Check sheet for the modelled part. Datum: model origin and axes. Units: mm. A direction names the side the tool comes from. Round coordinates to 2 decimals unless told otherwise and drop trailing zeros. Order: outer loops, then holes, each group sorted by start corner. A loop starts at its lowest first (then second) coordinate and runs counter-clockwise, first axis right, second up. Notation, with made-up numbers: (18, 47) -> (64, 47) arc R10 cw to (64, 66) -> close; hole circle Ø11 at (70.25, 52.5). An arc over 180 degrees is marked (long way). Answer in a Markdown table with one row per item.
```python
from build123d import *

# Parameters (mm, degrees)
F0_W     = 186
F0_H     = 44
F1_DEPTH = 15
F2_W     = 186
F2_H     = 44
F3_DEPTH = 2
F4_R     = 12
F5_SIZE  = 1.5


with BuildPart() as f1:
    # F0 (on Top) → F1 (new body)
    with BuildSketch(Plane.XY):
        with Locations((91, 20)):
            Rectangle(F0_W, F0_H)
        with BuildLine():
            ThreePointArc((122, 30), (124.9289321881, 37.0710678119), (132, 40))
            Line((132, 40), (172, 40))
            ThreePointArc((172, 40), (179.0710678119, 37.0710678119), (182, 30))
            Line((182, 30), (182, 10))
            ThreePointArc((182, 10), (179.0710678119, 2.9289321881), (172, 0))
            Line((172, 0), (132, 0))
            ThreePointArc((132, 0), (124.9289321881, 2.9289321881), (122, 10))
            Line((122, 10), (122, 30))
        make_face(mode=Mode.SUBTRACT)
        with BuildLine():
            Line((110, 0), (10, 0))
            ThreePointArc((10, 0), (2.9289321881, 2.9289321881), (0, 10))
            Line((0, 10), (0, 30))
            ThreePointArc((0, 30), (2.9289321881, 37.0710678119), (10, 40))
            Line((10, 40), (110, 40))
            ThreePointArc((110, 40), (117.0710678119, 37.0710678119), (120, 30))
            Line((120, 30), (120, 10))
            ThreePointArc((120, 10), (117.0710678119, 2.9289321881), (110, 0))
        make_face(mode=Mode.SUBTRACT)
    extrude(amount=F1_DEPTH)

    # F2 (on face) → F3 (join)
    with BuildSketch(Plane(origin=(0, 0, 0), x_dir=(1, 0, 0), z_dir=(0, 0, -1))):
        with Locations((91, -20)):
            Rectangle(F2_W, F2_H)
    extrude(amount=-F3_DEPTH)

    # F4
    f4_edges = [f1.edges().sort_by_distance(p)[0] for p in [
        (-2, -2, 7.5),
        (-2, 42, 7.5),
        (184, -2, 7.5),
        (184, 42, 7.5),
    ]]
    fillet(f4_edges, radius=F4_R)

    # F5
    f5_edges = [f1.edges().sort_by_distance(p)[0] for p in [
        (60, 0, 2),
        (117.071068, 2.928932, 2),
        (120, 20, 2),
        (117.071068, 37.071068, 2),
        (60, 40, 2),
        (2.928932, 37.071068, 2),
        (0, 20, 2),
        (2.928932, 2.928932, 2),
        (152, 0, 2),
        (179.071068, 2.928932, 2),
        (182, 20, 2),
        (179.071068, 37.071068, 2),
        (152, 40, 2),
        (124.928932, 37.071068, 2),
        (122, 20, 2),
        (124.928932, 2.928932, 2),
        (180.485281, 1.514719, 0),
    ]]
    chamfer(f5_edges, length=F5_SIZE)


solid = f1.part
```
(1) Scan lines: probe 1 along X at (y, z) = (10, 7.75); probe 2 along Y at (x, z) = (78.5, 10.25); probe 3 along X at (y, z) = (10.5, 3). Record each from-to range of solid material in increasing order. Write a range as from..to.
Solutions:
| item | result |
|---|---|
| probe 1 | -2..0, 120..122, 182..184 |
| probe 2 | -2..0, 40..42 |
| probe 3 | -2..0.5, 119.5..122.5, 181.5..184 |
(2) Depth check by flat-ended pin: pin 1 Ø18.5 at (x, y) = (73.5, 27.5) entering from +Z. Enter the tip coordinate at first touch or a pass-through.
Solutions:
| item | result |
|---|---|
| pin 1 | z = 2 |
(3) Section check C-C on x = 15.5. Record the boundary of the cut face in (y, z), plus the area to 3 significant figures.
Solutions:
| item | result |
|---|---|
| outline | (-2, 1.5) -> (-0.5, 0) -> (40.5, 0) -> (42, 1.5) -> (42, 15) -> (40, 15) -> (40, 3.5) -> (38.5, 2) -> (1.5, 2) -> (0, 3.5) -> (0, 15) -> (-2, 15) -> close |
| area | 140 mm^2 |
(4) Tool access check on faces 4 (the flat face through (-2, 20, 8)), 5 (the cylindrical face through (3.01, 2.85, 9.17)). Record the directions out of +Z, -Z, +X, -X, +Y, -Y that give a thin tool (end or side, any length) a straight path to the whole face; none if there is none.
Solutions:
| item | result |
|---|---|
| face 4 | +Z, -Z, -X, +Y, -Y |
| face 5 | +Z |
(5) Section check B-B on y = 14.5. Record the boundary of the cut face in (x, z).
Solutions:
| item | result |
|---|---|
| outline | (-2, 1.5) -> (-0.5, 0) -> (182.5, 0) -> (184, 1.5) -> (184, 15) -> (182, 15) -> (182, 3.5) -> (180.5, 2) -> (123.5, 2) -> (122, 3.5) -> (122, 15) -> (120, 15) -> (120, 3.5) -> (118.5, 2) -> (1.5, 2) -> (0, 3.5) -> (0, 15) -> (-2, 15) -> close |
(6) Section check A-A on z = 7.75. Record the boundary of the cut face in (x, y), plus the area to 3 significant figures.
Solutions:
| item | result |
|---|---|
| outline | (-2, 10) arc R12 ccw to (10, -2) -> (172, -2) arc R12 ccw to (184, 10) -> (184, 30) arc R12 ccw to (172, 42) -> (10, 42) arc R12 ccw to (-2, 30) -> close; hole (0, 10) arc R10 ccw to (10, 0) -> (110, 0) arc R10 ccw to (120, 10) -> (120, 30) arc R10 ccw to (110, 40) -> (10, 40) arc R10 ccw to (0, 30) -> close; hole (122, 10) arc R10 ccw to (132, 0) -> (172, 0) arc R10 ccw to (182, 10) -> (182, 30) arc R10 ccw to (172, 40) -> (132, 40) arc R10 ccw to (122, 30) -> close |
| area | 1,030 mm^2 |
(7) Draft check along X on faces 1 (the conical face through (125.9, 36.2, 2.2)), 2 (the flat face through (90, -2, 8)), 3 (the cylindrical face through (1.42, 38.39, 8.16)). Enter one of: pulls with the +X half, pulls with the -X half, needs draft (parallel to the pull), parting line crosses it, or undercut.
Solutions:
| item | result |
|---|---|
| face 1 | undercut |
| face 2 | needs draft |
| face 3 | pulls with the -X half |
